Work out the finished part from the listing and answer in its coordinate system (mm). A direction names the side the tool comes from. Coordinates: 2 decimals unless noted, no trailing zeros. Write each loop counter-clockwise with the first axis right and the second up, starting at its lowest first coordinate (ties: lowest second). Pieces come first, ordered by that corner, then holes. Notation, with made-up numbers: (-13.5, 88) - (4.5, 88) arc R20 ccw to (4.5, 127) - close; hole circle Ø4 at (67, 81.25). An arc over 180 degrees is marked (long way). One line per item, written item: value.
Autodesk Inventor part; units mm, degrees
ref_plane "Work Plane1" through (0, 4.6, -11) normal (0, 1, 0) x (-1, 0, 0)
ref_plane "YZ Plane" through (0, 0, 0) normal (1, 0, 0) x (0, 1, 0)
ref_plane "XY Plane" through (0, 0, 0) normal (0, 0, 1) x (1, 0, 0)
sketch "Sketch1" plane through (0, 0, 0) normal (0, 0, 1) x (1, 0, 0)
  circle A0 centre (0, 0) radius 5.1
  line L0 (-8.25, 8.25) -> (8.25, 8.25)
  line L1 (8.25, 8.25) -> (8.25, -8.25)
  line L2 (8.25, -8.25) -> (-8.25, -8.25)
  line L3 (-8.25, -8.25) -> (-8.25, 8.25)
  line L4 (-8.25, 8.25) -> (8.25, -8.25) construction
  line L5 (8.25, 8.25) -> (-8.25, -8.25) construction
  line L6 (0.75, -8.25) -> (-0.75, -8.25)
  line L7 (-0.75, -8.25) -> (-0.75, 8.25)
  line L8 (-0.75, 8.25) -> (0.75, 8.25)
  line L9 (0.75, 8.25) -> (0.75, -8.25)
  line L10 (0.75, -8.25) -> (-0.75, 8.25) construction
  line L11 (-0.75, -8.25) -> (0.75, 8.25) construction
  line L12 (8.25, 0.75) -> (-8.25, 0.75)
  line L13 (-8.25, 0.75) -> (-8.25, -0.75)
  line L14 (-8.25, -0.75) -> (8.25, -0.75)
  line L15 (8.25, -0.75) -> (8.25, 0.75)
  line L16 (8.25, 0.75) -> (-8.25, -0.75) construction
  line L17 (-8.25, 0.75) -> (8.25, -0.75) construction
  point P0 (0.75, -5.0446)
  point P1 (5.0446, -0.75)
  point P2 (5.0446, 0.75)
  point P3 (0.75, 5.0446)
  point P4 (-0.75, 5.0446)
  point P5 (-5.0446, 0.75)
  point P6 (-5.0446, -0.75)
  point P7 (-0.75, -5.0446)
  dimension "d0" = 10.2
  dimension "d1" = 16.5
  dimension "d2" = 1.5
  dimension "d3" = 1.5
  dimension "d38" = 16.5
extrude "Extrusion1" add sketch "Sketch1" against normal blind 11
extrude "Extrusion2" cut sketch "Sketch1" against normal blind 7 contours A0 L14 L9 L12 | A0 L12 L1 L14 | L12 L9 A0 | A0 L9 L14 | L9 L12 L7 A0 | A0 L7 L0 L9 | L9 L14 L7 L12 | L9 L2 L7 A0 | A0 L7 L14 L9 | L7 L12 A0 | L7 L14 A0 L12 | A0 L14 L7 | A0 L14 L3 L12
sketch "Sketch2" plane through (0, 0, -11) normal (0, 0, -1) x (-1, 0, 0)
  circle A0 centre (0, 0) radius 5
  dimension "d8" = 10
extrude "Extrusion3" [suppressed]
fillet "Fillet1" radius 6 4 edges at (8.25, 8.25, -5.5) (8.25, -8.25, -5.5) (-8.25, -8.25, -5.5) (-8.25, 8.25, -5.5)
sketch "Sketch3" plane through (0, 0, -26) normal (0, 0, -1) x (-1, 0, 0)
  line L0 (4, 2.7238) -> (10.2, 2.7238)
  line L1 (10.2, 2.7238) -> (10.2, -2.0551)
  line L2 (10.2, -2.0551) -> (4, -2.0551)
  line L3 (4, -2.0551) -> (4, 2.7238)
  arc A0 (2.5948, 0.1645) -> (2.1, -1.533) centre (0, 0) ccw
  circle A1 centre (0, 0) radius 5
  line L4 (0, 5) -> (10.2, 5)
  line L5 (10.2, 5) -> (10.2, -5)
  line L6 (10.2, -5) -> (0, -5)
  arc A2 (8.25, 2.25) -> (2.25, 8.25) centre (2.25, 2.25) ccw
  line L7 (2.25, 8.25) -> (-2.25, 8.25)
  arc A3 (-2.25, 8.25) -> (-8.25, 2.25) centre (-2.25, 2.25) ccw
  line L8 (-8.25, 2.25) -> (-8.25, -2.25)
  arc A4 (-8.25, -2.25) -> (-2.25, -8.25) centre (-2.25, -2.25) ccw
  line L9 (-2.25, -8.25) -> (2.25, -8.25)
  arc A5 (2.25, -8.25) -> (8.25, -2.25) centre (2.25, -2.25) ccw
  line L10 (8.25, -2.25) -> (8.25, 2.25)
  line L11 (-2.6, -2.9034) -> (-2.6, 2.8378)
  circle A6 centre (0, 0) radius 2.6
  point P0 (0.75, 5.0446)
  point P1 (2.1, -1.533)
  point P2 (2.5948, 0.1645)
  dimension "d12" = 6.2
  dimension "d13" = 4
  dimension "d14" = 5.2
extrude "Extrusion4" [suppressed]
sketch "Sketch4" plane through (-10.2, -5, -26) normal (-1, 0, 0) x (0, 0, 1)
  circle A0 centre (4, 5) radius 1.7
  line L0 (0, 0) -> (0, 10)
  point P0 (26, 5)
  point P1 (0, 5)
  point P2 (0, 5)
  dimension "d17" = 3.4
  dimension "d18" = 4
extrude "Extrusion5" [suppressed]
extrude "Extrusion6" [suppressed]
fillet "Fillet2" [suppressed]
fillet "Fillet3" [suppressed]
sketch "Sketch5" plane through (0, 0, -11) normal (0, 0, -1) x (-1, 0, 0)
  arc A0 (8.25, 2.25) -> (2.25, 8.25) centre (2.25, 2.25) ccw
  line L0 (2.25, 8.25) -> (-2.25, 8.25)
  arc A1 (-2.25, 8.25) -> (-8.25, 2.25) centre (-2.25, 2.25) ccw
  line L1 (-8.25, 2.25) -> (-8.25, -2.25)
  arc A2 (-8.25, -2.25) -> (-2.25, -8.25) centre (-2.25, -2.25) ccw
  line L2 (-2.25, -8.25) -> (2.25, -8.25)
  arc A3 (2.25, -8.25) -> (8.25, -2.25) centre (2.25, -2.25) ccw
  line L3 (8.25, -2.25) -> (8.25, 2.25)
  line L4 (-5.5, 5.5) -> (5.5, 5.5)
  line L5 (5.5, 5.5) -> (5.5, -5.5)
  line L6 (5.5, -5.5) -> (-5.5, -5.5)
  line L7 (-5.5, -5.5) -> (-5.5, 5.5)
  line L8 (-5.5, 5.5) -> (5.5, -5.5) construction
  line L9 (5.5, 5.5) -> (-5.5, -5.5) construction
  point P0 (0, 0)
  dimension "d31" = 11
  dimension "d32" = 11
extrude "Extrusion7" [suppressed]
sketch "Sketch6" plane through (0, 0, -7) normal (0, 0, 1) x (1, 0, 0)
  circle A0 centre (0, 0) radius 5.1
extrude "Extrusion8" cut sketch "Sketch6" against normal blind 2
sketch "Sketch7" plane through (0, 0, -11) normal (0, 0, -1) x (-1, 0, 0)
  circle A0 centre (0, 0) radius 4.6
  circle A1 centre (0, 0) radius 2.7
  dimension "d35" = 9.2
  dimension "d39" = 5.4
extrude "Extrusion9" add sketch "Sketch7" along normal blind 17.94
ref_plane "Work Plane1" through (0, 4.6, -11) normal (0, 1, 0) x (-1, 0, 0)
sketch "Sketch8" plane through (0, 4.6, -11) normal (0, 1, 0) x (-1, 0, 0)
  line L0 (2.7, -17.94) -> (-2.7, -17.94)
  line L1 (-2.7, -17.94) -> (-2.7, -14.94)
  line L2 (-2.7, -14.94) -> (2.7, -14.94)
  line L3 (2.7, -14.94) -> (2.7, -17.94)
  line L4 (-4.6, -17.94) -> (4.6, -17.94)
  point P0 (0, 11)
  point P1 (0, -17.94)
  dimension "d40" = 5.4
  dimension "d41" = 3
sketch "Sketch9" plane through (0, 0, -28.94) normal (0, 0, -1) x (-1, 0, 0)
  line L0 (2.7, 4.6) -> (-2.7, 4.6)
  line L1 (-2.7, 4.6) -> (2.7, 4.6)
  line L2 (2.7, 4.6) -> (2.7, 7.1)
  line L3 (2.7, 7.1) -> (-2.7, 7.1)
  line L4 (-2.7, 7.1) -> (-2.7, 4.6)
  line L5 (-4.2, 4.6) -> (4.2, 4.6)
  line L6 (4.2, 4.6) -> (4.2, 8.6)
  line L7 (4.2, 8.6) -> (-4.2, 8.6)
  line L8 (-4.2, 8.6) -> (-4.2, 4.6)
  line L9 (-4.2, 4.6) -> (-4.2, 1.8762)
  circle A0 centre (0, 0) radius 4.6
  line L10 (4.2, 4.6) -> (4.2, 1.8762)
  point P0 (0, 4.6)
  dimension "d42" = 5.4
  dimension "d43" = 2.5
  dimension "d44" = 1.5
  dimension "d45" = 1.5
  dimension "d46" = 1.5
extrude "Extrusion10" add sketch "Sketch9" against normal blind 4 contours L5 L10 A0 L0 | L2 L3 L4 L5 L8 L7 L6 | A0 L9 L5 L0
sketch "Sketch10" plane through (-4.2, 8.6, -28.94) normal (0, 1, 0) x (1, 0, 0)
  line L0 (4.2, -4) -> (4.2, 0)
  circle A0 centre (4.2, -2) radius 1.6
  point P0 (4.2, -28.94)
  dimension "d49" = 3.2
extrude "Extrusion11" cut sketch "Sketch10" against normal blind 9.25
properties part number "rubik_adapter"
Item 1: Section A-A, the plane x = -1.25 is taken. Give the number of separate pieces and of enclosed holes in the cut face, then the cut area to 3 significant figures.
Evaluation:
separate pieces: 4
enclosed holes: 0
area: 165 mm2
Item 2: Consider probe 1 along Y at (x, z) = (0, -24); probe 2 along Z at (x, y) = (1.75, -0.5); probe 3 along Z at (x, y) = (0, 3.55). Determine where each line is inside the solid, lowest interval first.
Evaluation:
probe 1: y = -4.6 to -2.7, 2.7 to 4.6
probe 2: z = -11 to -9
probe 3: z = -28.94 to -28.54, -25.34 to -9
Item 3: Which of the six approach directions +Z, -Z, +X, -X, +Y, -Y give full straight-line access (tool end or side, diameter ignored) to faces 1 (the face through (4.2, 5, -27)), 2 (the face through (-2.47, -3.88, -19.84)), 3 (the face through (-7, 0.75, -3)), 4 (the face through (0.75, 7, -3)), 5 (the face through (-4.2, 5, -27))?
Evaluation:
face 1: -Z, +X, +Y
face 2: none
face 3: +Z, +X, -X
face 4: +Z, +Y, -Y
face 5: -Z, -X, +Y
Item 4: Determine the mould class of faces 6 (the face through (-7, 0, -7)), 7 (the face through (-0.75, -7, -3)), 8 (the face through (0, 0, -11)), 9 (the face through (-6.539, 6.446, -5.577)) for opening direction Y: +Y half, -Y half, draft (parallel to the pull), parting line (faces both ways), or undercut.
Evaluation:
face 6: undercut
face 7: draft
face 8: undercut
face 9: +Y half
Item 5: Section D-D, the plane x = -3.25 is taken. Determine the outline of the cut face in (y, z).
Evaluation:
outline: (-8.17, -11) - (-3.26, -11) - (-3.26, -28.94) - (8.6, -28.94) - (8.6, -24.94) - (3.26, -24.94) - (3.26, -11) - (8.17, -11) - (8.17, 0) - (3.93, 0) - (3.93, -9) - (-3.93, -9) - (-3.93, 0) - (-8.17, 0) - close
Item 6: Section B-B, the plane z = -21 is taken. Determine the outline of the cut face in (x, y).
Evaluation:
outline: circle Ø9.2 at (0, 0); hole circle Ø5.4 at (0, 0)
Item 7: Section C-C, the plane y = 0 is taken. Determine the outline of the cut face in (x, z), then the cut area to 3 significant figures.
Evaluation:
outline: (-8.25, -11) - (-4.6, -11) - (-4.6, -28.94) - (-2.7, -28.94) - (-2.7, -11) - (2.7, -11) - (2.7, -28.94) - (4.6, -28.94) - (4.6, -11) - (8.25, -11) - (8.25, -7) - (5.1, -7) - (5.1, -9) - (-5.1, -9) - (-5.1, -7) - (-8.25, -7) - close
area: 114 mm2
Item 8: Given pin 1 (1.9 mm diameter, centred on x = 0, z = -26.94, fed in from -Y); pin 2 (1 mm diameter, centred on x = -1, z = -6, fed in from +Y); pin 3 (4 mm diameter, centred on y = 2, z = -20.5, fed in from -X), each flat-ended and moving along its own axis, determine where each tip first touches the part or whether it passes through.
Evaluation:
pin 1: stops at y = -4.6
pin 2: stops at y = 8.25
pin 3: stops at x = -4.6
